For this review, take the finished solid that the model builds, in its own axes (mm). Give positions to 0.01 mm unless a question says otherwise; leave off trailing zeros. Loops run counter-clockwise (first coordinate to the right, second up) from the corner with the lowest first, then second, coordinate; pieces in that order, holes last. Notation, with made-up numbers: (36, 41) - (81, 41) arc R9 cw to (81, 48) - close; hole circle Ø7 at (83.25, -34). An arc over 180 degrees is marked (long way). Put each result on its own line as item: value.
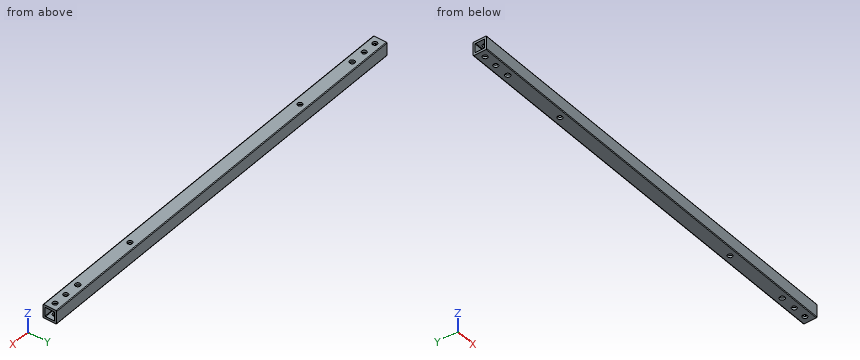
from build123d import *

# Parameters (mm, degrees)
BOSS_EXTRUDE1_DEPTH              = 295.91
F_1_4_CLEARANCE_HOLE1_AT_2_COUNT = 2
F_1_4_CLEARANCE_HOLE1_AT_2_PITCH = 31.75
F_1_4_CLEARANCE_HOLE1_AT_3_COUNT = 2
F_1_4_CLEARANCE_HOLE1_AT_3_PITCH = 50.8
F_1_4_CLEARANCE_HOLE1_AT_4_COUNT = 2
F_1_4_CLEARANCE_HOLE1_AT_4_PITCH = 165.735
F_1_4_CLEARANCE_HOLE2_D          = 7.14248


with BuildPart() as part:
    # Sketch4 → Boss-Extrude1 (new, symmetric)
    with BuildSketch(Plane(origin=(0, 0, 0), x_dir=(0, 0, -1), z_dir=(1, 0, 0))):
        with BuildLine():
            Line((9.525, -8.5725), (9.525, 8.5725))
            ThreePointArc((9.525, 8.5725), (9.246019209, 9.246019209), (8.5725, 9.525))
            Line((8.5725, 9.525), (-8.5725, 9.525))
            ThreePointArc((-8.5725, 9.525), (-9.246019209, 9.246019209), (-9.525, 8.5725))
            Line((-9.525, 8.5725), (-9.525, -8.5725))
            ThreePointArc((-9.525, -8.5725), (-9.246019209, -9.246019209), (-8.5725, -9.525))
            Line((-8.5725, -9.525), (8.5725, -9.525))
            ThreePointArc((8.5725, -9.525), (9.246019209, -9.246019209), (9.525, -8.5725))
        make_face()
        with BuildLine():
            Line((6.477, 5.8293), (6.477, -5.8293))
            ThreePointArc((6.477, -5.8293), (6.287293062, -6.287293062), (5.8293, -6.477))
            Line((5.8293, -6.477), (-5.8293, -6.477))
            ThreePointArc((-5.8293, -6.477), (-6.287293062, -6.287293062), (-6.477, -5.8293))
            Line((-6.477, -5.8293), (-6.477, 5.8293))
            ThreePointArc((-6.477, 5.8293), (-6.287293062, 6.287293062), (-5.8293, 6.477))
            Line((-5.8293, 6.477), (5.8293, 6.477))
            ThreePointArc((5.8293, 6.477), (6.287293062, 6.287293062), (6.477, 5.8293))
        make_face(mode=Mode.SUBTRACT)
    extrude(amount=BOSS_EXTRUDE1_DEPTH, both=True)

    # Sketch6 → 1/4 Clearance Hole1 (revolve, cut)
    with BuildSketch(Plane(origin=(318.135, 0, -9.525), x_dir=(0, 1, 0), z_dir=(1, 0, 0))):
        Polygon((0, 0), (0, 21.079827343), (3.3782, 19.05), (3.3782, 0), align=None)
    f_1_4_clearance_hole1 = revolve(axis=Axis((318.135, 0, -15.875), (0, 0, 1)), mode=Mode.SUBTRACT)

    # 1/4 Clearance Hole1 at 2: 1/4 Clearance Hole1 ×2
    with Locations(*[(-i * F_1_4_CLEARANCE_HOLE1_AT_2_PITCH, 0, 0) for i in range(1, F_1_4_CLEARANCE_HOLE1_AT_2_COUNT)]):
        add(f_1_4_clearance_hole1, mode=Mode.SUBTRACT)

    # 1/4 Clearance Hole1 at 3: 1/4 Clearance Hole1 ×2
    with Locations(*[(-i * F_1_4_CLEARANCE_HOLE1_AT_3_PITCH, 0, 0) for i in range(1, F_1_4_CLEARANCE_HOLE1_AT_3_COUNT)]):
        add(f_1_4_clearance_hole1, mode=Mode.SUBTRACT)

    # 1/4 Clearance Hole1 at 4: 1/4 Clearance Hole1 ×2
    with Locations(*[(-i * F_1_4_CLEARANCE_HOLE1_AT_4_PITCH, 0, 0) for i in range(1, F_1_4_CLEARANCE_HOLE1_AT_4_COUNT)]):
        add(f_1_4_clearance_hole1, mode=Mode.SUBTRACT)

    # Mirror2: 1/4 Clearance Hole1 across plane
    add(f_1_4_clearance_hole1.mirror(Plane(origin=(0, 0, 0), x_dir=(0, 0, 1), z_dir=(1, 0, 0))), mode=Mode.SUBTRACT)

    # Mirror2 copy 1 sketch → Mirror2 copy 1 (revolve, cut)
    with BuildSketch(Plane(origin=(-286.385, 0, -9.525), x_dir=(0, 1, 0), z_dir=(-1, 0, 0))):
        Polygon((0, 0), (0, -21.079827343), (3.3782, -19.05), (3.3782, 0), align=None)
    revolve(axis=Axis((-286.385, 0, -15.875), (0, 0, -1)), mode=Mode.SUBTRACT)

    # Mirror2 copy 2 sketch → Mirror2 copy 2 (revolve, cut)
    with BuildSketch(Plane(origin=(-267.335, 0, -9.525), x_dir=(0, 1, 0), z_dir=(-1, 0, 0))):
        Polygon((0, 0), (0, -21.079827343), (3.3782, -19.05), (3.3782, 0), align=None)
    revolve(axis=Axis((-267.335, 0, -15.875), (0, 0, -1)), mode=Mode.SUBTRACT)

    # Mirror2 copy 3 sketch → Mirror2 copy 3 (revolve, cut)
    with BuildSketch(Plane(origin=(-152.4, 0, -9.525), x_dir=(0, 1, 0), z_dir=(-1, 0, 0))):
        Polygon((0, 0), (0, -21.079827343), (3.3782, -19.05), (3.3782, 0), align=None)
    revolve(axis=Axis((-152.4, 0, -15.875), (0, 0, -1)), mode=Mode.SUBTRACT)

    # 1/4 Clearance Hole2 (through all)
    with Locations(Plane.XY.offset(9.525)):
        with Locations((245.745, 0), (-245.745, 0)):
            Hole(F_1_4_CLEARANCE_HOLE2_D / 2)


solid = part.part
1) Wall thickness on line 1 (Y direction, x = -194, z = 2.75) (3 decimals); line 2 (Y direction, x = -152.4, z = 7.15) (3 decimals): over which ranges is each line inside the solid? List them lowest first.
Geometry check:
line 1: y = -9.525 to -6.477, 6.477 to 9.525
line 2: y = -9.525 to -3.378, 3.378 to 9.525
2) Take a section at A-A on z = 0.25. State the section outline as (x, y) points (3 decimals).
Geometry check:
outline: (-295.91, -9.525) - (295.91, -9.525) - (295.91, -6.477) - (-295.91, -6.477) - close; (-295.91, 6.477) - (295.91, 6.477) - (295.91, 9.525) - (-295.91, 9.525) - close
3) Take a section at C-C on y = 0. State how many separate pieces and enclosed holes the cut face has, and give its area (3 significant figures).
Geometry check:
separate pieces: 18
enclosed holes: 0
area: 3,270 mm²
4) Insertion check: pin 1 Ø8 at (x, y) = (152.4, 0) entering from +Z (3 decimals). The pin has a flat end and moves straight along its axis. Give the tip position at first contact, or say it passes through.
Geometry check:
pin 1: stops at z = 9.525
5) Take a section at B-B on x = 104. State the section outline as (y, z) points (1 decimal).
Geometry check:
outline: (-9.5, -8.6) arc R1 ccw to (-8.6, -9.5) - (8.6, -9.5) arc R1 ccw to (9.5, -8.6) - (9.5, 8.6) arc R1 ccw to (8.6, 9.5) - (-8.6, 9.5) arc R1 ccw to (-9.5, 8.6) - close; hole (-6.5, -5.8) arc R0.6 ccw to (-5.8, -6.5) - (5.8, -6.5) arc R0.6 ccw to (6.5, -5.8) - (6.5, 5.8) arc R0.6 ccw to (5.8, 6.5) - (-5.8, 6.5) arc R0.6 ccw to (-6.5, 5.8) - close
